Design review of the part built by this model. Coordinates are the model's own, in mm. Round coordinates to 2 decimals unless told otherwise and drop trailing zeros. Loops run counter-clockwise (first coordinate to the right, second up) from the corner with the lowest first, then second, coordinate; pieces in that order, holes last. Notation, with made-up numbers: (38.5, -1.5) - (80.5, -1.5) arc R15 cw to (80.5, 24.5) - close; hole circle Ø3 at (48.5, 73.5). An arc over 180 degrees is marked (long way). One line per question, with ' | ' between items. Start each with the question number.
from build123d import *

# Parameters (mm, degrees)
SKETCH1_W           = 140
SKETCH1_H           = 20
BOSS_EXTRUDE1_DEPTH = 2
SKETCH2_R           = 2
CUT_EXTRUDE1_DEPTH  = 3
CUT_EXTRUDE2_REACH  = 4
SKETCH3_R           = 3.5


with BuildPart() as part:
    # Sketch1 → Boss-Extrude1 (new body)
    with BuildSketch(Plane.XY):
        Rectangle(SKETCH1_W, SKETCH1_H)
    extrude(amount=BOSS_EXTRUDE1_DEPTH)

    # Sketch2 → Cut-Extrude1 (cut, through all)
    with BuildSketch(Plane.XY.offset(2)):
        with Locations((-60, 0)):
            Circle(SKETCH2_R)
        with Locations((60, 0)):
            Circle(SKETCH2_R)
    extrude(amount=-CUT_EXTRUDE1_DEPTH, mode=Mode.SUBTRACT)

    # Sketch3 → Cut-Extrude2 (cut, up to next)
    with BuildSketch(Plane.XY.offset(2), mode=Mode.PRIVATE) as cut_extrude2_sk1:
        with Locations((22, 0)):
            Circle(SKETCH3_R)
    cut_extrude2_tool1 = extrude(cut_extrude2_sk1.sketch, amount=-CUT_EXTRUDE2_REACH, mode=Mode.PRIVATE) & part.part
    add(cut_extrude2_tool1.solids().sort_by_distance((22, 0, 2))[0], mode=Mode.SUBTRACT)
    # Sketch3 → Cut-Extrude2 (cut, up to next)
    with BuildSketch(Plane.XY.offset(2), mode=Mode.PRIVATE) as cut_extrude2_sk2:
        with Locations((-22, 0)):
            Circle(SKETCH3_R)
    cut_extrude2_tool2 = extrude(cut_extrude2_sk2.sketch, amount=-CUT_EXTRUDE2_REACH, mode=Mode.PRIVATE) & part.part
    add(cut_extrude2_tool2.solids().sort_by_distance((-22, 0, 2))[0], mode=Mode.SUBTRACT)


solid = part.part
1. The part is to be moulded in two halves that separate along Y. For faces 1 (the face through (-1, 0, 0)), 2 (the face through (25.34, 1.05, 1.01)), say which applies: pulls with the +Y half, pulls with the -Y half, needs draft (parallel to the pull), parting line crosses it, or undercut.
2. Take a section at B-B, the plane x = -22. Give the boundary of the cut face in (y, z), then the cut area to 3 significant figures.
3. Clearance check with flat-ended pins moving along their axes: P1, Ø3, axis at x = 60, y = 0, coming from the -Z side; P2, Ø5, axis at x = -4.5, y = 2.5, coming from the -Z side. State where each tip first meets the part, or that it passes through.
4. To check wall thickness, follow line 1 along Y through (x, z) = (-22, 0.5); line 2 along Y through (x, z) = (-60, 0.8). State the ranges of each line that lie inside material, in increasing order.
5. Take a section at D-D, the plane x = 60. Give the boundary of the cut face in (y, z).
6. Take a section at C-C, the plane z = 0.5. Give the boundary of the cut face in (x, y).
7. Take a section at A-A, the plane y = 0. Give the boundary of the cut face in (x, z), then the cut area to 3 significant figures.
Answer list:
1) face 1: needs draft | face 2: undercut
2) outline: (-10, 0) - (-3.5, 0) - (-3.5, 2) - (-10, 2) - close; (3.5, 0) - (10, 0) - (10, 2) - (3.5, 2) - close | area: 26.0 mm²
3) P1: passes through | P2: stops at z = 0
4) line 1: y = -10 to -3.5, 3.5 to 10 | line 2: y = -10 to -2, 2 to 10
5) outline: (-10, 0) - (-2, 0) - (-2, 2) - (-10, 2) - close; (2, 0) - (10, 0) - (10, 2) - (2, 2) - close
6) outline: (-70, -10) - (70, -10) - (70, 10) - (-70, 10) - close; hole circle Ø4 at (-60, 0); hole circle Ø7 at (-22, 0); hole circle Ø7 at (22, 0); hole circle Ø4 at (60, 0)
7) outline: (-70, 0) - (-62, 0) - (-62, 2) - (-70, 2) - close; (-58, 0) - (-25.5, 0) - (-25.5, 2) - (-58, 2) - close; (-18.5, 0) - (18.5, 0) - (18.5, 2) - (-18.5, 2) - close; (25.5, 0) - (58, 0) - (58, 2) - (25.5, 2) - close; (62, 0) - (70, 0) - (70, 2) - (62, 2) - close | area: 236 mm²
